Verification items for the finished model (mm, model axes). Face numbers are marked on the shaded views. A direction names the side the tool comes from. Round coordinates to 2 decimals unless told otherwise and drop trailing zeros. Order: outer loops, then holes, each group sorted by start corner. A loop starts at its lowest first (then second) coordinate and runs counter-clockwise, first axis right, second up.
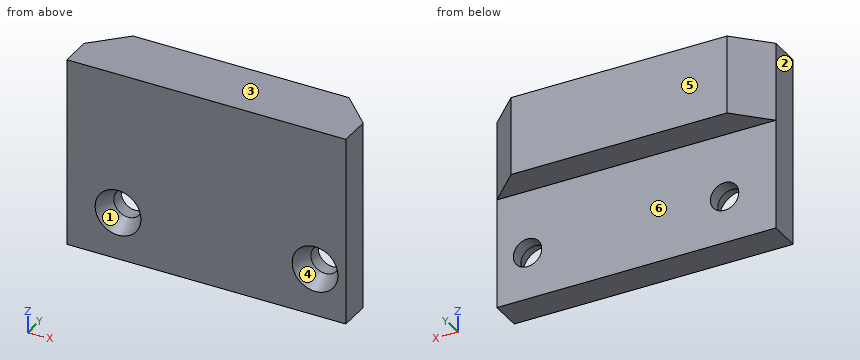
```python
from build123d import *

# Parameters (mm, degrees)
BOX054_W                = 35.4
BOX054_H                = 8
BOX054_DEPTH            = 10
CHAMFER005_SIZE         = 4
CYLINDER109_R           = 1.8
CYLINDER109_DEPTH       = 10
BODY054_PLACEMENT_ANGLE = 90
ARRAY001047_Y_COUNT     = 2
ARRAY001047_Y_PITCH     = 25
ARRAY001047_Z_COUNT     = 3
ARRAY001047_Z_PITCH     = 20
BODY055_PLACEMENT_ANGLE = 90
BOX053_W                = 35.4
BOX053_H                = 4
BOX053_DEPTH            = 24


with BuildPart() as chamfer005:
    # Box054 → Box054 (new body)
    with BuildSketch(Plane(origin=(-17.7, -21.8, 0), x_dir=(1, 0, 0), z_dir=(0, 0, 1))):
        with Locations((17.7, 4)):
            Rectangle(BOX054_W, BOX054_H)
    extrude(amount=BOX054_DEPTH)

    # Chamfer005
    chamfer005_edges = [chamfer005.edges().sort_by_distance(p)[0] for p in [
        (-17.7, -13.8, 5),
        (17.7, -13.8, 5),
    ]]
    chamfer(chamfer005_edges, length=CHAMFER005_SIZE)


with BuildPart() as cone:
    # Cone → Cone (revolve)
    with BuildSketch(Plane(origin=(0, 0, 7.5), x_dir=(1, 0, 0), z_dir=(0, -1, 0))):
        Polygon((0, 0), (1.8, 0), (3, 2.5), (0, 2.5), align=None)
    revolve(axis=Axis((0, 0, 7.5), (0, 0, 1)))


with BuildPart() as top_screw_hole_array_clone:
    # Cylinder109 → Cylinder109 (new body)
    with BuildSketch(Plane.XY):
        Circle(CYLINDER109_R)
    extrude(amount=CYLINDER109_DEPTH)

    # Fusion085: union Cone
    add(cone.part)


with BuildPart() as top_screw_hole_array_clone_1:
    # Body054 placement: moved
    add(top_screw_hole_array_clone.part.rotate(Axis((0, 0, 0), (0, -1, 0)), BODY054_PLACEMENT_ANGLE))

    # Array001047 Y: top screw hole array clone ×2


with BuildPart() as top_screw_hole_array_clone_2:
    add(top_screw_hole_array_clone_1.part)
    with Locations(*[(0, i * ARRAY001047_Y_PITCH, 0) for i in range(1, ARRAY001047_Y_COUNT)]):
        add(top_screw_hole_array_clone_1.part)

    # Array001047 Z: top screw hole array clone ×3


with BuildPart() as top_screw_hole_array_clone_3:
    add(top_screw_hole_array_clone_2.part)
    with Locations(*[(0, 0, i * ARRAY001047_Z_PITCH) for i in range(1, ARRAY001047_Z_COUNT)]):
        add(top_screw_hole_array_clone_2.part)


with BuildPart() as top_screw_hole_array_clone_4:
    # Array001047 placement: moved
    add(top_screw_hole_array_clone_3.part.moved(Location((0, 4, 35))))


with BuildPart() as top_screw_hole_array_clone_5:
    # Body055 placement: moved
    add(top_screw_hole_array_clone_4.part.moved(Location((17.8, -12, -83))).rotate(Axis((17.8, -12, -83), (0, 0, 1)), BODY055_PLACEMENT_ANGLE))


with BuildPart() as fusion084:
    # Box053 → Box053 (new body)
    with BuildSketch(Plane(origin=(-17.7, -21.8, -14), x_dir=(1, 0, 0), z_dir=(0, 0, 1))):
        with Locations((17.7, 2)):
            Rectangle(BOX053_W, BOX053_H)
    extrude(amount=BOX053_DEPTH)

    # Cut023020: cut top screw hole array clone
    add(top_screw_hole_array_clone_5.part, mode=Mode.SUBTRACT)

    # Fusion084: union Chamfer005
    add(chamfer005.part)


solid = fusion084.part
```
1) Sectioned sample at B-B on z = -8. Record the cut outline in (x, y).
2) Sectioned sample at A-A on x = -11.2. Record the cut outline in (y, z).
3) Scan lines: probe 1 along X at (y, z) = (-18.25, -8); probe 2 along Z at (x, y) = (13.8, -18.6); probe 3 along X at (y, z) = (-21.25, -10.25). Record each from-to range of solid material in increasing order.
4) Go/stop test with flat-tipped pins: pin 1 Ø1.2 at (x, y) = (6.5, -15.5) entering from -Z; pin 2 Ø11 at (x, z) = (-8, -8) entering from +Y; pin 3 Ø2 at (x, z) = (-11.2, -8) entering from -Y. Record where each tip stops, or that it passes through.
5) Tool access check on the marked faces 5 and 6. Record the directions out of +Z, -Z, +X, -X, +Y, -Y that give a thin tool (end or side, any length) a straight path to the whole face; none if there is none.
6) Sectioned sample at C-C on z = 3.5. Record the cut outline in (x, y).
7) Sectioned sample at D-D on x = -2. Record the cut outline in (y, z).
8) Draft check along Z on the marked faces 1, 2, 3 and 4. Enter one of: released by +Z, released by -Z, zero draft, split by the parting line, or undercut.
Returned:
1. outline: (-17.7, -21.8) - (-14.1, -21.8) - (-13, -19.5) - (-13, -17.8) - (-17.7, -17.8) - close; (-9.4, -19.5) - (-8.3, -21.8) - (10.9, -21.8) - (12, -19.5) - (12, -17.8) - (-9.4, -17.8) - close; (15.6, -19.5) - (16.7, -21.8) - (17.7, -21.8) - (17.7, -17.8) - (15.6, -17.8) - close
2. outline: (-21.8, -14) - (-17.8, -14) - (-17.8, -9.8) - (-19.5, -9.8) - (-21.8, -10.9) - close; (-21.8, -5.1) - (-19.5, -6.2) - (-17.8, -6.2) - (-17.8, 0) - (-13.8, 0) - (-13.8, 10) - (-21.8, 10) - close
3. probe 1: x = -17.7 to -13, -9.4 to 12, 15.6 to 17.7
3. probe 2: z = -14 to -9.8, -6.2 to 10
3. probe 3: x = -17.7 to -12.58, -9.82 to 12.42, 15.18 to 17.7
4. pin 1: stops at z = 0
4. pin 2: stops at y = -17.8
4. pin 3: passes through
5. face 5: +Z, -Z, +X, -X, +Y
5. face 6: -Z, +X, -X, +Y
6. outline: (-17.7, -21.8) - (17.7, -21.8) - (17.7, -17.8) - (13.7, -13.8) - (-13.7, -13.8) - (-17.7, -17.8) - close
7. outline: (-21.8, -14) - (-17.8, -14) - (-17.8, 0) - (-13.8, 0) - (-13.8, 10) - (-21.8, 10) - close
8. face 1: undercut
8. face 2: zero draft
8. face 3: released by +Z
8. face 4: undercut
